```python
from build123d import *

# Parameters (mm, degrees)
CYLINDER007_R          = 1.6
CYLINDER007_DEPTH      = 10
CYLINDER006_R          = 1.6
CYLINDER006_DEPTH      = 10
CYLINDER005_R          = 1.6
CYLINDER005_DEPTH      = 10
CYLINDER004_R          = 1.6
CYLINDER004_DEPTH      = 10
CYLINDER_R             = 1.6
CYLINDER_DEPTH         = 50
CYLINDER_ROLL_ANGLE    = 90
BOX024_W               = 6
BOX024_H               = 3
BOX024_DEPTH           = 10
BOX023_W               = 6
BOX023_H               = 3
BOX023_DEPTH           = 10
BOX021_W               = 6
BOX021_H               = 3
BOX021_DEPTH           = 3
BOX022_W               = 13
BOX022_H               = 34
BOX022_DEPTH           = 3
CYLINDER003_R          = 1.6
CYLINDER003_DEPTH      = 10
CYLINDER002_R          = 1.6
CYLINDER002_DEPTH      = 10
BOX019_W               = 45
BOX019_H               = 56
BOX019_DEPTH           = 3
BOX018_W               = 10
BOX018_H               = 10
BOX018_DEPTH           = 23
BOX018_PITCH_ANGLE     = 9
BOX013_W               = 8.6
BOX013_H               = 10
BOX013_DEPTH           = 17.8
BOX017_W               = 10
BOX017_H               = 8
BOX017_DEPTH           = 23
BOX017_PITCH_ANGLE     = 9
BOX012_W               = 8.6
BOX012_H               = 8
BOX012_DEPTH           = 17.8
BOX016_W               = 10
BOX016_H               = 10
BOX016_DEPTH           = 23
BOX016_PITCH_ANGLE     = 9
BOX011_W               = 8.6
BOX011_H               = 10
BOX011_DEPTH           = 17.8
BOX008_W               = 10
BOX008_H               = 34
BOX008_DEPTH           = 23
BOX008_PITCH_ANGLE     = -9
BOX007_W               = 8.6
BOX007_H               = 34
BOX007_DEPTH           = 17.8
BOX006_W               = 4
BOX006_H               = 40
BOX006_DEPTH           = 3
BOX006_PLACEMENT_ANGLE = 30
BOX004_W               = 10
BOX004_H               = 40
BOX004_DEPTH           = 19
BOX004_PITCH_ANGLE     = 9
BOX005_W               = 2.8
BOX005_H               = 40
BOX005_DEPTH           = 2.8
BOX005_PITCH_ANGLE     = 45
BOX003_W               = 7
BOX003_H               = 40
BOX003_DEPTH           = 19
BOX003_PITCH_ANGLE     = -9
BOX001_W               = 10.5
BOX001_H               = 40
BOX001_DEPTH           = 20
BOX_W                  = 34
BOX_H                  = 40
BOX_DEPTH              = 42
BOX020_W               = 6
BOX020_H               = 3
BOX020_DEPTH           = 3


with BuildPart() as cylinder007:
    # Cylinder007 → Cylinder007 (new body)
    with BuildSketch(Plane(origin=(28, 44, 0), x_dir=(1, 0, 0), z_dir=(0, 0, 1))):
        Circle(CYLINDER007_R)
    extrude(amount=CYLINDER007_DEPTH)


with BuildPart() as cylinder006:
    # Cylinder006 → Cylinder006 (new body)
    with BuildSketch(Plane(origin=(5, 44, 0), x_dir=(1, 0, 0), z_dir=(0, 0, 1))):
        Circle(CYLINDER006_R)
    extrude(amount=CYLINDER006_DEPTH)


with BuildPart() as cylinder005:
    # Cylinder005 → Cylinder005 (new body)
    with BuildSketch(Plane(origin=(28, -4, 0), x_dir=(1, 0, 0), z_dir=(0, 0, 1))):
        Circle(CYLINDER005_R)
    extrude(amount=CYLINDER005_DEPTH)


with BuildPart() as cylinder004:
    # Cylinder004 → Cylinder004 (new body)
    with BuildSketch(Plane(origin=(5, -4, 0), x_dir=(1, 0, 0), z_dir=(0, 0, 1))):
        Circle(CYLINDER004_R)
    extrude(amount=CYLINDER004_DEPTH)


with BuildPart() as cylinder:
    # Cylinder → Cylinder (new body)
    with BuildSketch(Plane.XY):
        Circle(CYLINDER_R)
    extrude(amount=CYLINDER_DEPTH)


with BuildPart() as cylinder_1:
    # Cylinder roll: moved
    add(cylinder.part.rotate(Axis((0, 0, 0), (1, 0, 0)), CYLINDER_ROLL_ANGLE))


with BuildPart() as cylinder_2:
    # Cylinder placement: moved
    add(cylinder_1.part.moved(Location((-1, 45, 5))))


with BuildPart() as cube024:
    # Box024 → Box024 (new body)
    with BuildSketch(Plane(origin=(-6, 37, 3), x_dir=(1, 0, 0), z_dir=(0, 0, 1))):
        with Locations((3, 1.5)):
            Rectangle(BOX024_W, BOX024_H)
    extrude(amount=BOX024_DEPTH)


with BuildPart() as cube023:
    # Box023 → Box023 (new body)
    with BuildSketch(Plane(origin=(-6, 0, 3), x_dir=(1, 0, 0), z_dir=(0, 0, 1))):
        with Locations((3, 1.5)):
            Rectangle(BOX023_W, BOX023_H)
    extrude(amount=BOX023_DEPTH)


with BuildPart() as cube021:
    # Box021 → Box021 (new body)
    with BuildSketch(Plane(origin=(28, 37, 42), x_dir=(1, 0, 0), z_dir=(0, 0, 1))):
        with Locations((3, 1.5)):
            Rectangle(BOX021_W, BOX021_H)
    extrude(amount=BOX021_DEPTH)


with BuildPart() as cube022:
    # Box022 → Box022 (new body)
    with BuildSketch(Plane(origin=(-6.6, 3, 0), x_dir=(1, 0, 0), z_dir=(0, 0, 1))):
        with Locations((6.5, 17)):
            Rectangle(BOX022_W, BOX022_H)
    extrude(amount=BOX022_DEPTH)


with BuildPart() as cylinder003:
    # Cylinder003 → Cylinder003 (new body)
    with BuildSketch(Plane(origin=(34, 32, 0), x_dir=(1, 0, 0), z_dir=(0, 0, 1))):
        Circle(CYLINDER003_R)
    extrude(amount=CYLINDER003_DEPTH)


with BuildPart() as cylinder002:
    # Cylinder002 → Cylinder002 (new body)
    with BuildSketch(Plane(origin=(34, 8, 0), x_dir=(1, 0, 0), z_dir=(0, 0, 1))):
        Circle(CYLINDER002_R)
    extrude(amount=CYLINDER002_DEPTH)


with BuildPart() as cube019:
    # Box019 → Box019 (new body)
    with BuildSketch(Plane(origin=(-6, -8, 0), x_dir=(1, 0, 0), z_dir=(0, 0, 1))):
        with Locations((22.5, 28)):
            Rectangle(BOX019_W, BOX019_H)
    extrude(amount=BOX019_DEPTH)


with BuildPart() as cube018:
    # Box018 → Box018 (new body)
    with BuildSketch(Plane.XY):
        with Locations((5, 5)):
            Rectangle(BOX018_W, BOX018_H)
    extrude(amount=BOX018_DEPTH)


with BuildPart() as cube018_1:
    # Box018 pitch: moved
    add(cube018.part.rotate(Axis((0, 0, 0), (0, 1, 0)), BOX018_PITCH_ANGLE))


with BuildPart() as cube018_2:
    # Box018 placement: moved
    add(cube018_1.part.moved(Location((27.6, 3, 20.8))))


with BuildPart() as cube013:
    # Box013 → Box013 (new body)
    with BuildSketch(Plane(origin=(27.6, 3, 3), x_dir=(1, 0, 0), z_dir=(0, 0, 1))):
        with Locations((4.3, 5)):
            Rectangle(BOX013_W, BOX013_H)
    extrude(amount=BOX013_DEPTH)


with BuildPart() as cube017:
    # Box017 → Box017 (new body)
    with BuildSketch(Plane.XY):
        with Locations((5, 4)):
            Rectangle(BOX017_W, BOX017_H)
    extrude(amount=BOX017_DEPTH)


with BuildPart() as cube017_1:
    # Box017 pitch: moved
    add(cube017.part.rotate(Axis((0, 0, 0), (0, 1, 0)), BOX017_PITCH_ANGLE))


with BuildPart() as cube017_2:
    # Box017 placement: moved
    add(cube017_1.part.moved(Location((27.6, 16, 20.8))))


with BuildPart() as cube012:
    # Box012 → Box012 (new body)
    with BuildSketch(Plane(origin=(27.6, 16, 3), x_dir=(1, 0, 0), z_dir=(0, 0, 1))):
        with Locations((4.3, 4)):
            Rectangle(BOX012_W, BOX012_H)
    extrude(amount=BOX012_DEPTH)


with BuildPart() as cube016:
    # Box016 → Box016 (new body)
    with BuildSketch(Plane.XY):
        with Locations((5, 5)):
            Rectangle(BOX016_W, BOX016_H)
    extrude(amount=BOX016_DEPTH)


with BuildPart() as cube016_1:
    # Box016 pitch: moved
    add(cube016.part.rotate(Axis((0, 0, 0), (0, 1, 0)), BOX016_PITCH_ANGLE))


with BuildPart() as cube016_2:
    # Box016 placement: moved
    add(cube016_1.part.moved(Location((27.6, 27, 20.8))))


with BuildPart() as cube011:
    # Box011 → Box011 (new body)
    with BuildSketch(Plane(origin=(27.6, 27, 3), x_dir=(1, 0, 0), z_dir=(0, 0, 1))):
        with Locations((4.3, 5)):
            Rectangle(BOX011_W, BOX011_H)
    extrude(amount=BOX011_DEPTH)


with BuildPart() as cube008:
    # Box008 → Box008 (new body)
    with BuildSketch(Plane.XY):
        with Locations((5, 17)):
            Rectangle(BOX008_W, BOX008_H)
    extrude(amount=BOX008_DEPTH)


with BuildPart() as cube008_1:
    # Box008 pitch: moved
    add(cube008.part.rotate(Axis((0, 0, 0), (0, 1, 0)), BOX008_PITCH_ANGLE))


with BuildPart() as cube008_2:
    # Box008 placement: moved
    add(cube008_1.part.moved(Location((-3.3, 3, 18.2))))


with BuildPart() as cube007:
    # Box007 → Box007 (new body)
    with BuildSketch(Plane(origin=(-2.19, 3, 3), x_dir=(1, 0, 0), z_dir=(0, 0, 1))):
        with Locations((4.3, 17)):
            Rectangle(BOX007_W, BOX007_H)
    extrude(amount=BOX007_DEPTH)


with BuildPart() as cube006:
    # Box006 → Box006 (new body)
    with BuildSketch(Plane.XY):
        with Locations((2, 20)):
            Rectangle(BOX006_W, BOX006_H)
    extrude(amount=BOX006_DEPTH)


with BuildPart() as cube006_1:
    # Box006 placement: moved
    add(cube006.part.moved(Location((21.6, 0, 22))).rotate(Axis((21.6, 0, 22), (0, -1, 0)), BOX006_PLACEMENT_ANGLE))


with BuildPart() as cube004:
    # Box004 → Box004 (new body)
    with BuildSketch(Plane.XY):
        with Locations((5, 20)):
            Rectangle(BOX004_W, BOX004_H)
    extrude(amount=BOX004_DEPTH)


with BuildPart() as cube004_1:
    # Box004 pitch: moved
    add(cube004.part.rotate(Axis((0, 0, 0), (0, 1, 0)), BOX004_PITCH_ANGLE))


with BuildPart() as cube004_2:
    # Box004 placement: moved
    add(cube004_1.part.moved(Location((15.3, 0, 25.6))))


with BuildPart() as cube005:
    # Box005 → Box005 (new body)
    with BuildSketch(Plane.XY):
        with Locations((1.4, 20)):
            Rectangle(BOX005_W, BOX005_H)
    extrude(amount=BOX005_DEPTH)


with BuildPart() as cube005_1:
    # Box005 pitch: moved
    add(cube005.part.rotate(Axis((0, 0, 0), (0, 1, 0)), BOX005_PITCH_ANGLE))


with BuildPart() as cube005_2:
    # Box005 placement: moved
    add(cube005_1.part.moved(Location((9.1, 0, 24))))


with BuildPart() as cube003:
    # Box003 → Box003 (new body)
    with BuildSketch(Plane.XY):
        with Locations((3.5, 20)):
            Rectangle(BOX003_W, BOX003_H)
    extrude(amount=BOX003_DEPTH)


with BuildPart() as cube003_1:
    # Box003 pitch: moved
    add(cube003.part.rotate(Axis((0, 0, 0), (0, 1, 0)), BOX003_PITCH_ANGLE))


with BuildPart() as cube003_2:
    # Box003 placement: moved
    add(cube003_1.part.moved(Location((9, 0, 24))))


with BuildPart() as cube001:
    # Box001 → Box001 (new body)
    with BuildSketch(Plane(origin=(11.15, 0, 22), x_dir=(1, 0, 0), z_dir=(0, 0, 1))):
        with Locations((5.25, 20)):
            Rectangle(BOX001_W, BOX001_H)
    extrude(amount=BOX001_DEPTH)


with BuildPart() as cut021:
    # Box → Box (new body)
    with BuildSketch(Plane.XY):
        with Locations((17, 20)):
            Rectangle(BOX_W, BOX_H)
    extrude(amount=BOX_DEPTH)

    # Cut: cut Cube001
    add(cube001.part, mode=Mode.SUBTRACT)

    # Cut001: cut Cube003
    add(cube003_2.part, mode=Mode.SUBTRACT)

    # Cut002: cut Cube005
    add(cube005_2.part, mode=Mode.SUBTRACT)

    # Cut003: cut Cube004
    add(cube004_2.part, mode=Mode.SUBTRACT)

    # Cut004: cut Cube006
    add(cube006_1.part, mode=Mode.SUBTRACT)

    # Cut005: cut Cube007
    add(cube007.part, mode=Mode.SUBTRACT)

    # Cut006: cut Cube008
    add(cube008_2.part, mode=Mode.SUBTRACT)

    # Cut011: cut Cube011
    add(cube011.part, mode=Mode.SUBTRACT)

    # Cut012: cut Cube016
    add(cube016_2.part, mode=Mode.SUBTRACT)

    # Cut013: cut Cube012
    add(cube012.part, mode=Mode.SUBTRACT)

    # Cut014: cut Cube017
    add(cube017_2.part, mode=Mode.SUBTRACT)

    # Cut015: cut Cube013
    add(cube013.part, mode=Mode.SUBTRACT)

    # Cut016: cut Cube018
    add(cube018_2.part, mode=Mode.SUBTRACT)

    # Fusion: union Cube019
    add(cube019.part)

    # Cut019: cut Cylinder002
    add(cylinder002.part, mode=Mode.SUBTRACT)

    # Cut020: cut Cylinder003
    add(cylinder003.part, mode=Mode.SUBTRACT)

    # Cut021: cut Cube022
    add(cube022.part, mode=Mode.SUBTRACT)


with BuildPart() as cut026:
    # Box020 → Box020 (new body)
    with BuildSketch(Plane(origin=(28, 0, 42), x_dir=(1, 0, 0), z_dir=(0, 0, 1))):
        with Locations((3, 1.5)):
            Rectangle(BOX020_W, BOX020_H)
    extrude(amount=BOX020_DEPTH)

    # Fusion001: union Cut021
    add(cut021.part)

    # Fusion002: union Cube021
    add(cube021.part)

    # Fusion003: union Cube023
    add(cube023.part)

    # Fusion004: union Cube024
    add(cube024.part)

    # Cut022: cut Cylinder
    add(cylinder_2.part, mode=Mode.SUBTRACT)

    # Cut023: cut Cylinder004
    add(cylinder004.part, mode=Mode.SUBTRACT)

    # Cut024: cut Cylinder005
    add(cylinder005.part, mode=Mode.SUBTRACT)

    # Cut025: cut Cylinder006
    add(cylinder006.part, mode=Mode.SUBTRACT)

    # Cut026: cut Cylinder007
    add(cylinder007.part, mode=Mode.SUBTRACT)


solid = cut026.part
```
Here's how the part is built. I have some questions about the finished solid (model axes, mm). A direction names the side the tool comes from. Round coordinates to 2 decimals unless told otherwise and drop trailing zeros. Write each loop counter-clockwise with the first axis right and the second up, starting at its lowest first coordinate (ties: lowest second). Pieces come first, ordered by that corner, then holes.
Q1. If we mould it in two halves opening along X, with no side actions, what happens to faces 1 (the flat face through (26.58, 19.72, 32.89)), 2 (the flat face through (2, 3, 16)), 3 (the flat face through (29.255, 31.93, 31.252))? For each: +X half, -X half, draft (parallel to the pull), parting line (faces both ways), or undercut.
Q2. Which directions (+Z, -Z, +X, -X, +Y, -Y) give clear straight access to the entire face, cutting with the end or side of a thin tool? Please do faces 4 (the flat face through (6.4, 20, 1)), 5 (the flat face through (28, 1, 43)), 6 (the flat face through (14, 40, 19)), 7 (the flat face through (31, 3, 24)), 8 (the flat face through (23.33, 20.28, 23)).
Q3. If we section it at A-A on x = -1: Write out the boundary of the cut face in (y, z).
Q4. If we section it at D-D on y = 44: Write out the boundary of the cut face in (x, z), plus the area to 3 significant figures.
Q5. Will these pins go through, and if not, where does the flat tip stop? P1, Ø3.5, axis at x = -3, y = 1, coming from the +Z side; P2, Ø0.9, axis at y = 16, z = 1.5, coming from the -X side; P3, Ø3, axis at y = 6, z = 10, coming from the +X side; P4, Ø1, axis at x = 19, y = 28.5, coming from the -Z side.
Q6. Please list where these lines run through material, in increasing order: probe 1 along Y at (x, z) = (28, 1); probe 2 along X at (y, z) = (44, 1.2); probe 3 along Y at (x, z) = (5, 1).
Q7. If we section it at C-C on z = 15: Write out the boundary of the cut face in (x, y), plus the area to 3 significant figures.
Answer below:
1. face 1: undercut
1. face 2: draft
1. face 3: +X half
2. face 4: -Z, -X
2. face 5: +Z, -X, +Y, -Y
2. face 6: +Z, +X, -X, +Y
2. face 7: +X
2. face 8: +Z, +Y, -Y
3. outline: (-8, 0) - (3, 0) - (3, 3.4) - (0, 3.4) - (0, 3) - (-8, 3) - close; (0, 6.6) - (3, 6.6) - (3, 13) - (0, 13) - close; (37, 0) - (48, 0) - (48, 3) - (40, 3) - (40, 3.4) - (37, 3.4) - close; (37, 6.6) - (40, 6.6) - (40, 13) - (37, 13) - close
4. outline: (-6, 0) - (3.4, 0) - (3.4, 3) - (-6, 3) - close; (6.6, 0) - (26.4, 0) - (26.4, 3) - (6.6, 3) - close; (29.6, 0) - (39, 0) - (39, 3) - (29.6, 3) - close
4. area: 116 mm2
5. P1: stops at z = 13
5. P2: stops at x = 6.4
5. P3: stops at x = 27.6
5. P4: stops at z = 0
6. probe 1: y = -8 to -5.6, -2.4 to 42.4, 45.6 to 48
6. probe 2: x = -6 to 3.4, 6.6 to 26.4, 29.6 to 39
6. probe 3: y = -8 to -5.6, -2.4 to 3, 37 to 42.4, 45.6 to 48
7. outline: (0, 0) - (34, 0) - (34, 3) - (27.6, 3) - (27.6, 13) - (34, 13) - (34, 16) - (27.6, 16) - (27.6, 24) - (34, 24) - (34, 27) - (27.6, 27) - (27.6, 37) - (34, 37) - (34, 40) - (0, 40) - (0, 37) - (6.41, 37) - (6.41, 3) - (0, 3) - close
7. area: 963 mm2
